Source: three-view drawing plus pictorial views. Frame: mm from the lowest corner of the part. A direction names the side the tool comes from. Give positions to 0.01 mm unless a question says otherwise; leave off trailing zeros. Order: outer loops, then holes, each group sorted by start corner. A loop starts at its lowest first (then second) coordinate and runs counter-clockwise, first axis right, second up. Notation, with made-up numbers: M -25.75,-28.5 L -13.75,-28.5 A16 cw -13.75,-14.5 Z; hole C 81.5,5 d5. An arc over 180 degrees is marked long. One line per question, with ' | ' between items. Start each with the question number.
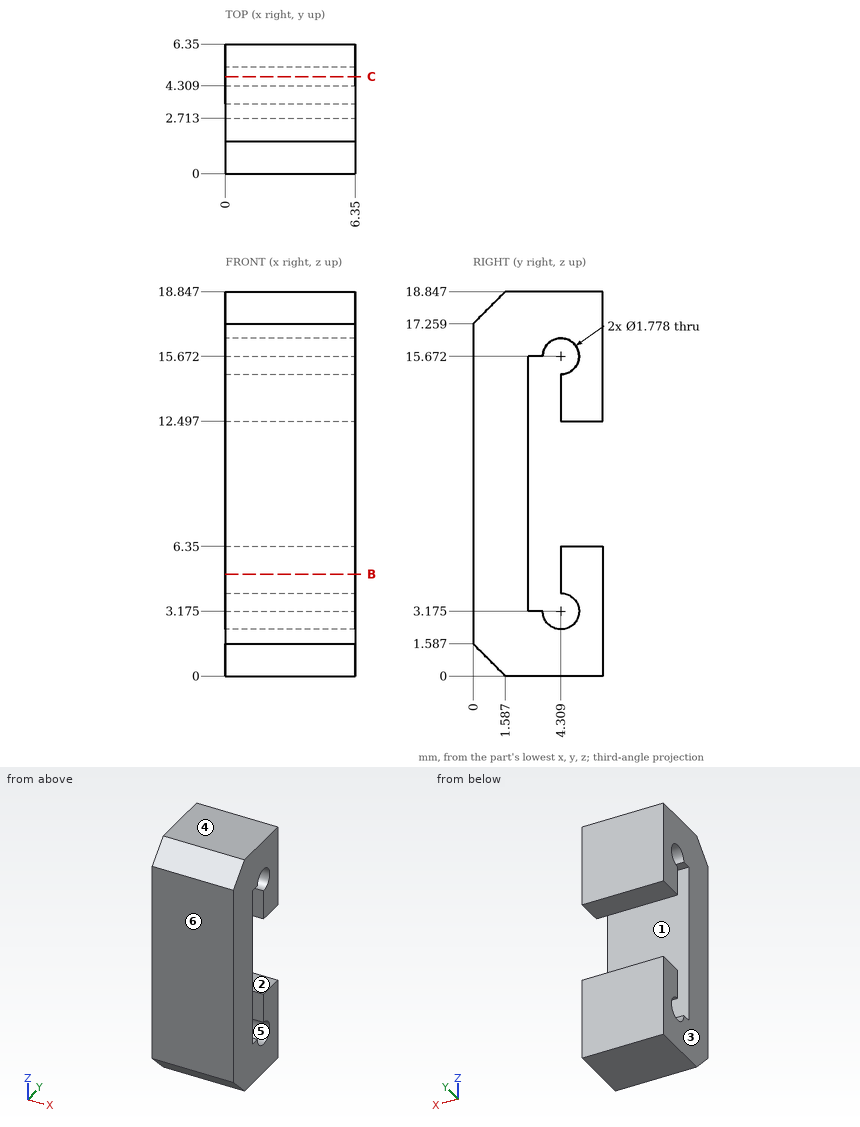
Item 1: Cut plane B-B on z = 5. Return the cut outline in (x, y).
Item 2: Mould query, pull axis Y, two halves, no side actions, for the marked faces 4, 5 and 6. Classes: pulls with the +Y half, pulls with the -Y half, needs draft (parallel to the pull), parting line crosses it, or undercut.
Item 3: Pin query (flat end, axial travel): pin 1 Ø1.1 at (y, z) = (4.31, 3.18) entering from -X. Return the tip coordinate at first contact, or that it passes through.
Item 4: Reachability of the marked faces 1, 2 and 3 from +Z, -Z, +X, -X, +Y, -Y: full face, straight path, thin tool, end or side. Return the list, or none.
Item 5: Line query: line 1 (Y direction, x = 3.25, z = 13.75); line 2 (Z direction, x = 1, y = 3) (1 decimal); line 3 (Z direction, x = 0.5, y = 5.25). Output: solid intervals per line, ascending.
Item 6: Cut plane C-C on y = 4.75. Return the cut outline in (x, z).
Results are:
1) outline: M 0,0 L 6.35,0 L 6.35,2.71 L 0,2.71 Z; M 0,4.31 L 6.35,4.31 L 6.35,6.35 L 0,6.35 Z
2) face 4: needs draft | face 5: undercut | face 6: pulls with the -Y half
3) pin 1: passes through
4) face 1: +X, -X | face 2: +X, -X, +Y | face 3: +Z, -Z, -X, +Y, -Y
5) line 1: y = 0 to 2.71, 4.31 to 6.35 | line 2: z = 0 to 3.2, 15.7 to 18.8 | line 3: z = 0 to 6.35, 12.5 to 18.85
6) outline: M 0,0 L 6.35,0 L 6.35,2.4 L 0,2.4 Z; M 0,3.95 L 6.35,3.95 L 6.35,6.35 L 0,6.35 Z; M 0,12.5 L 6.35,12.5 L 6.35,14.9 L 0,14.9 Z; M 0,16.44 L 6.35,16.44 L 6.35,18.85 L 0,18.85 Z
